```python
from build123d import *

# Parameters (mm, degrees)
F1_DEPTH = 1
F2_W     = 2
F2_H     = 8
F3_DEPTH = 1
F4_R     = 0.5
F5_W     = 2.2095986642
F5_H     = 7.0855088998
F6_DEPTH = 5
F7_R     = 1


with BuildPart() as f1:
    # F0 (on Top) → F1 (new body)
    with BuildSketch(Plane.XY):
        with BuildLine():
            ThreePointArc((-2.6457513111, 3), (4, 0), (-2.6457513111, -3))
            Line((-2.6457513111, -3), (-4.0599648734, -4.4142135624))
            Line((-4.0599648734, -4.4142135624), (-2.4741784358, -6))
            Line((-2.4741784358, -6), (15.9400351266, -6))
            Line((15.9400351266, -6), (15.9400351266, 6))
            Line((15.9400351266, 6), (-2.4741784358, 6))
            Line((-2.4741784358, 6), (-4.0599648734, 4.4142135624))
            Line((-4.0599648734, 4.4142135624), (-2.6457513111, 3))
        make_face()
    extrude(amount=F1_DEPTH)

    # F2 (on face) → F3 (join)
    with BuildSketch(Plane.XY.offset(1)):
        with Locations((11.9400351266, 0)):
            Rectangle(F2_W, F2_H)
    extrude(amount=F3_DEPTH)

    # F4
    f4_edges = [f1.edges().sort_by_distance(p)[0] for p in [
        (-2.645751, -3, 0.5),
        (-2.645751, 3, 0.5),
        (-4.059965, -4.414214, 0.5),
        (-2.474178, -6, 0.5),
        (-4.059965, 4.414214, 0.5),
        (-2.474178, 6, 0.5),
        (10.940035, -4, 1.5),
        (12.940035, -4, 1.5),
        (10.940035, 4, 1.5),
        (12.940035, 4, 1.5),
        (15.940035, 6, 0.5),
        (15.940035, -6, 0.5),
    ]]
    fillet(f4_edges, radius=F4_R)

    # F5 (on face) → F6 (join)
    with BuildSketch(Plane.XY.offset(1)):
        with Locations((8.1892169546, 0.1541808015)):
            Rectangle(F5_W, F5_H)
    extrude(amount=F6_DEPTH)

    # F7
    f7_edges = [f1.edges().sort_by_distance(p)[0] for p in [
        (8.189217, 3.696935, 6),
        (7.084418, 0.154181, 6),
        (8.189217, -3.388574, 6),
        (9.294016, 0.154181, 6),
    ]]
    fillet(f7_edges, radius=F7_R)


solid = f1.part
```
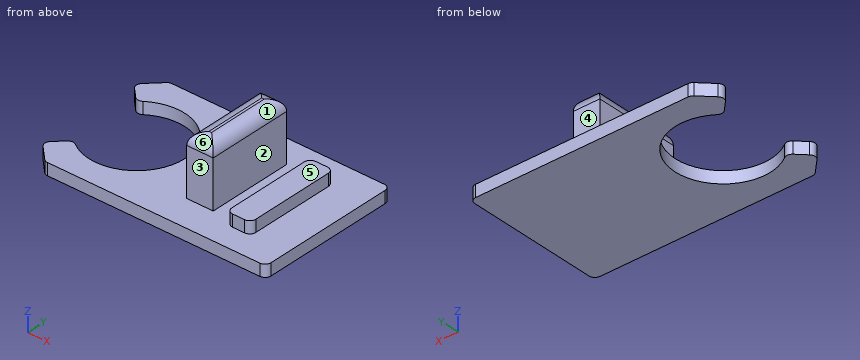
Model file for the job. Use its own axes, mm. Face numbers are marked on the shaded views. A direction names the side the tool comes from. Give positions to 0.01 mm unless a question says otherwise; leave off trailing zeros. Loops run counter-clockwise (first coordinate to the right, second up) from the corner with the lowest first, then second, coordinate; pieces in that order, holes last. Notation, with made-up numbers: M -6.75,39 L -2.75,39 A14 cw -2.75,63 Z; hole C -32.75,73 d10. An arc over 180 degrees is marked long. Use one line per item in the form item = value.
Item 1: Slice it at A-A on x = 0. List the corners of the cut face in (y, z).
Filled in:
outline = M -6,0 L -4,0 L -4,1 L -6,1 Z; M 4,0 L 6,0 L 6,1 L 4,1 Z
Item 2: Slice it at C-C on y = 0. List the corners of the cut face in (x, z), and give its area (3 significant figures).
Filled in:
outline = M 4,0 L 15.94,0 L 15.94,1 L 12.94,1 L 12.94,2 L 10.94,2 L 10.94,1 L 9.29,1 L 9.29,5 A1 ccw 8.29,6 L 8.08,6 A1 ccw 7.08,5 L 7.08,1 L 4,1 Z
area = 24.6 mm^2
Item 3: Which spindle directions (+Z, -Z, +X, -X, +Y, -Y) get a long thin tool onto all of the face, cutting with end or side? Do the marked faces 4, 5 and 6. Say none if no direction does.
Filled in:
face_4 = +Z, -X, +Y
face_5 = +Z, +X, +Y, -Y
face_6 = +Z, +X, -X, -Y
Item 4: Flat gauge pins, fed straight in: pin 1 Ø3 at (x, y) = (12.5, 1.5) entering from +Z; pin 2 Ø1.1 at (y, z) = (0.5, 1.5) entering from -X; pin 3 Ø3 at (x, z) = (5.5, 3) entering from +Y; pin 4 Ø1.1 at (x, z) = (12, 1.5) entering from +Y. Where does each tip first touch, or does it go through?
Filled in:
pin_1 = 2
pin_2 = 3.93
pin_3 = through
pin_4 = 6
Item 5: Two-plate mould, pull along X, no slides. Class the marked faces 1, 2 and 3: released by +X, released by -X, zero draft, split by the parting line, or undercut.
Filled in:
face_1 = released by +X
face_2 = undercut
face_3 = zero draft
Item 6: Slice it at D-D on x = 8.75. List the corners of the cut face in (y, z), and give its area (3 significant figures).
Filled in:
outline = M -6,0 L 6,0 L 6,1 L 3.7,1 L 3.7,5 A1 ccw 3.15,5.89 L -2.84,5.89 A1 ccw -3.39,5 L -3.39,1 L -6,1 Z
area = 46.4 mm^2
Item 7: Slice it at B-B on z = 1.25. List the corners of the cut face in (x, y).
Filled in:
outline = M 7.08,-3.39 L 9.29,-3.39 L 9.29,3.7 L 7.08,3.7 Z; M 10.94,-3.5 A0.5 ccw 11.44,-4 L 12.44,-4 A0.5 ccw 12.94,-3.5 L 12.94,3.5 A0.5 ccw 12.44,4 L 11.44,4 A0.5 ccw 10.94,3.5 Z
Item 8: Drill centre lines: L1, parallel to Y at x = 0, z = 0.7; L2, parallel to X at y = 2.25, z = 1.2; L3, parallel to Z at x = 13.5, y = 5.5. Where is each one in solid material? Low to high.
Filled in:
L1 = -6 to -4, 4 to 6
L2 = 7.08 to 9.29, 10.94 to 12.94
L3 = 0 to 1
